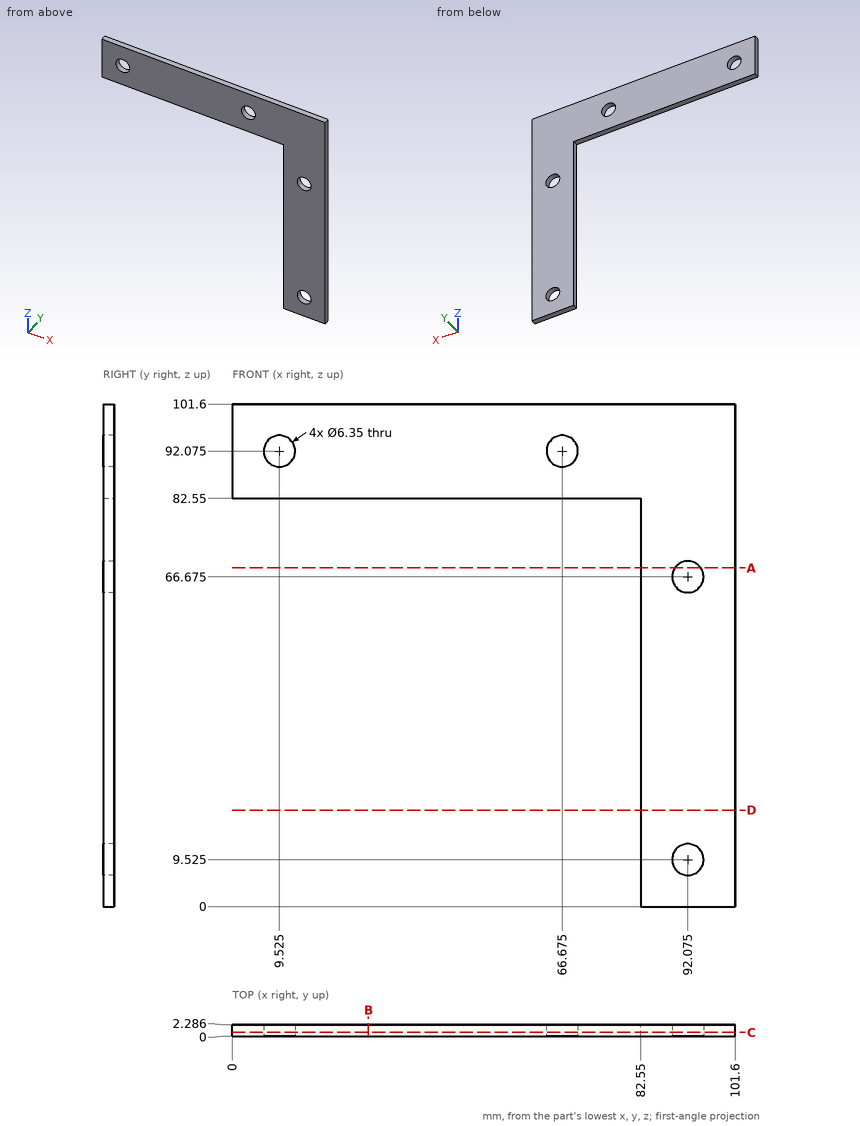
Print and shaded views of the part. All mm, measured from the part's lowest x, y and z. Give positions to 0.01 mm unless a question says otherwise; leave off trailing zeros. Loops run counter-clockwise (first coordinate to the right, second up) from the corner with the lowest first, then second, coordinate; pieces in that order, holes last. Notation, with made-up numbers: (-8.75, -38) -> (37.25, -38) arc R25 ccw to (37.25, -16) -> close; hole circle Ø5 at (57, 88). An arc over 180 degrees is marked (long way). Answer in a Markdown table with one row per item.
Item 1: Slice it at C-C on y = 0.75. Write the cut outline in (x, z) (3 decimals), plus the area to 3 significant figures.
Findings below:
| item | result |
|---|---|
| outline | (0, 82.55) -> (82.55, 82.55) -> (82.55, 0) -> (101.6, 0) -> (101.6, 101.6) -> (0, 101.6) -> close; hole circle Ø6.35 at (9.525, 92.075); hole circle Ø6.35 at (66.675, 92.075); hole circle Ø6.35 at (92.075, 9.525); hole circle Ø6.35 at (92.075, 66.675) |
| area | 3,380 mm² |
Item 2: Slice it at D-D on z = 19.5. Write the cut outline in (x, y).
Findings below:
| item | result |
|---|---|
| outline | (82.55, 0) -> (101.6, 0) -> (101.6, 2.29) -> (82.55, 2.29) -> close |
Item 3: Flat gauge pins, fed straight in: P1, Ø1, axis at y = 1, z = 36.5, coming from the -X side; P2, Ø5, axis at x = 92.075, z = 9.525, coming from the +Y side; P3, Ø0.7, axis at x = 31.5, y = 1, coming from the -Z side. Where does each tip first touch, or does it go through?
Findings below:
| item | result |
|---|---|
| P1 | stops at x = 82.55 |
| P2 | passes through |
| P3 | stops at z = 82.55 |
Item 4: Slice it at A-A on z = 68.5. Write the cut outline in (x, y), plus the area to 3 significant figures.
Findings below:
| item | result |
|---|---|
| outline | (82.55, 0) -> (89.48, 0) -> (89.48, 2.29) -> (82.55, 2.29) -> close; (94.67, 0) -> (101.6, 0) -> (101.6, 2.29) -> (94.67, 2.29) -> close |
| area | 31.7 mm² |
Item 5: Slice it at B-B on x = 27.5. Write the cut outline in (y, z).
Findings below:
| item | result |
|---|---|
| outline | (0, 82.55) -> (2.29, 82.55) -> (2.29, 101.6) -> (0, 101.6) -> close |
Item 6: Probe line 1 along X through (y, z) = (1.6, 60); line 2 along Z through (x, y) = (68, 0.85). List the from-to ranges inside material, lowest first. Write a range as [from, to].
Findings below:
| item | result |
|---|---|
| line 1 | x = [82.55, 101.6] |
| line 2 | z = [82.55, 89.19], [94.96, 101.6] |
